from build123d import *

# Parameters (mm, degrees)
SKETCH1_W           = 300
SKETCH1_H           = 150
BOSS_EXTRUDE1_DEPTH = 5
SKETCH3_W           = 300
SKETCH3_H           = 150
SKETCH3_W_2         = 290
SKETCH3_H_2         = 140
BOSS_EXTRUDE2_DEPTH = 100
SKETCH4_W           = 290
SKETCH4_H           = 50
SKETCH4_H_2         = 60
BOSS_EXTRUDE3_DEPTH = 10
SKETCH7_R           = 12
CUT_EXTRUDE1_DEPTH  = 351
FILLET1_R           = 20
SKETCH10_W          = 180
SKETCH10_H          = 30
BOSS_EXTRUDE4_DEPTH = 15
SKETCH11_W          = 180
SKETCH11_H          = 30
BOSS_EXTRUDE5_DEPTH = 25
CHAMFER2_SIZE       = 15
CHAMFER3_SIZE       = 25
SKETCH12_W          = 133.404446906
SKETCH12_H          = 15
CUT_EXTRUDE2_DEPTH  = 50


with BuildPart() as part:
    # Sketch1 → Boss-Extrude1 (new body)
    with BuildSketch(Plane(origin=(0, 0, 0), x_dir=(1, 0, 0), z_dir=(0, 1, 0))):
        with Locations((150, 75)):
            Rectangle(SKETCH1_W, SKETCH1_H)
    extrude(amount=BOSS_EXTRUDE1_DEPTH)

    # Sketch3 → Boss-Extrude2 (add)
    with BuildSketch(Plane(origin=(0, 5, 0), x_dir=(1, 0, 0), z_dir=(0, 1, 0))):
        with Locations((150, 75)):
            Rectangle(SKETCH3_W, SKETCH3_H)
        with Locations((150, 75)):
            Rectangle(SKETCH3_W_2, SKETCH3_H_2, mode=Mode.SUBTRACT)
    extrude(amount=BOSS_EXTRUDE2_DEPTH)

    # Sketch4 → Boss-Extrude3 (add)
    with BuildSketch(Plane(origin=(0, 5, 0), x_dir=(1, 0, 0), z_dir=(0, 1, 0))):
        with Locations((150, 120)):
            Rectangle(SKETCH4_W, SKETCH4_H)
        with Locations((150, 35)):
            Rectangle(SKETCH4_W, SKETCH4_H_2)
    extrude(amount=BOSS_EXTRUDE3_DEPTH)

    # Sketch7 → Cut-Extrude1 (cut, through all)
    with BuildSketch(Plane(origin=(0, 5, 0), x_dir=(1, 0, 0), z_dir=(0, 1, 0))):
        with Locations(Location((150, 80, 0), (0, 0, 270))):
            Circle(SKETCH7_R)
    extrude(amount=-CUT_EXTRUDE1_DEPTH, mode=Mode.SUBTRACT)

    # Fillet1
    fillet1_edges = [part.edges().sort_by_distance(p)[0] for p in [
        (5, 60, -145),
        (5, 60, -5),
        (295, 60, -5),
        (295, 60, -145),
        (0, 52.5, -150),
        (300, 52.5, -150),
        (300, 52.5, 0),
        (0, 52.5, 0),
    ]]
    fillet(fillet1_edges, radius=FILLET1_R)

    # Sketch10 → Boss-Extrude4 (add)
    with BuildSketch(Plane.XY.offset(-145)):
        with Locations((150, 90)):
            Rectangle(SKETCH10_W, SKETCH10_H)
    extrude(amount=BOSS_EXTRUDE4_DEPTH)

    # Sketch11 → Boss-Extrude5 (add)
    with BuildSketch(Plane(origin=(0, 0, -5), x_dir=(-1, 0, 0), z_dir=(0, 0, -1))):
        with Locations((-150, 90)):
            Rectangle(SKETCH11_W, SKETCH11_H)
    extrude(amount=BOSS_EXTRUDE5_DEPTH)

    # Chamfer2
    chamfer2_edges = [part.edges().sort_by_distance(p)[0] for p in [
        (240, 90, -145),
        (150, 75, -145),
        (60, 90, -145),
    ]]
    chamfer(chamfer2_edges, length=CHAMFER2_SIZE - 0.0001)  # a hair under: the kernel refuses the full size

    # Chamfer3
    chamfer3_edges = [part.edges().sort_by_distance(p)[0] for p in [
        (60, 90, -5),
        (150, 75, -5),
        (240, 90, -5),
    ]]
    chamfer(chamfer3_edges, length=CHAMFER3_SIZE - 0.0001)  # a hair under: the kernel refuses the full size

    # Sketch12 → Cut-Extrude2 (cut)
    with BuildSketch(Plane(origin=(0, 105, 0), x_dir=(1, 0, 0), z_dir=(0, 1, 0))):
        with Locations((150, 7.5)):
            Rectangle(SKETCH12_W, SKETCH12_H)
    extrude(amount=-CUT_EXTRUDE2_DEPTH, mode=Mode.SUBTRACT)


solid = part.part
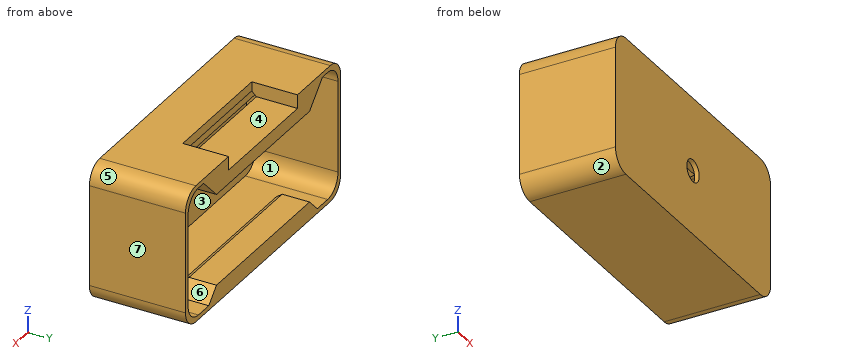
Source: CAD feature listing. Evaluate the final solid. Frame: model axes, mm. Face numbers are marked on the shaded views. A direction names the side the tool comes from. Round coordinates to 2 decimals unless told otherwise and drop trailing zeros. Write each loop counter-clockwise with the first axis right and the second up, starting at its lowest first coordinate (ties: lowest second). Pieces come first, ordered by that corner, then holes. Notation, with made-up numbers: (-20.75, 86.5) - (-2.75, 86.5) arc R7 cw to (-2.75, 98.5) - close; hole circle Ø3 at (-15.5, 40). An arc over 180 degrees is marked (long way). Use CSV: the item, a comma, the result in double quotes. Start each with the question number.
(1) Cut plane D-D, the plane y = 63.5. Return loops of the section in (x, z).
(2) Cut plane C-C, the plane z = -115. Return loops of the section in (x, y), and give its area (3 significant figures).
(3) First-contact query: pin 1 Ø22.5 at (x, y) = (131, 77.5) entering from +Z; pin 2 Ø25 at (x, z) = (102, -112.5) entering from +Y; pin 3 Ø4.5 at (y, z) = (86.5, -9) entering from +X. Flat tips, straight axial feed; report the tip coordinate or a pass-through.
(4) Mould query, pull axis Z, two halves, no side actions, for the marked faces 5, 6 and 7. Classes: pulls with the +Z half, pulls with the -Z half, needs draft (parallel to the pull), parting line crosses it, or undercut.
(5) Set-up query: the marked faces 1, 2, 3 and 4. Return all of +Z, -Z, +X, -X, +Y, -Y with unobstructed straight access to the full face (end or side cutting, diameter ignored); none if empty.
(6) Material intervals for probe 1 along Z at (x, y) = (92, 11.5); probe 2 along X at (y, z) = (98.5, -52); probe 3 along Z at (x, y) = (222, 88.5), sorted ascending. Write a range as [from, to].
(7) Cut plane A-A, the plane z = -80. Return loops of the section in (x, y), and give its area (3 significant figures).
(8) Cut plane B-B, the plane x = 150. Give the number of separate pieces and of enclosed holes in the cut face, and give its area (3 significant figures).
Geometry says:
1,outline,"(0, -130) arc R20 ccw to (20, -150) - (280, -150) arc R20 ccw to (300, -130) - (300, -20) arc R20 ccw to (280, 0) - (216.7, 0) - (216.7, -15) - (83.3, -15) - (83.3, 0) - (20, 0) arc R20 ccw to (0, -20) - close; hole (5, -125) arc R20 ccw to (25, -145) - (45, -145) - (48.5, -141.5) - (251.5, -141.5) - (255, -145) - (275, -145) arc R20 ccw to (295, -125) - (295, -25) arc R20 ccw to (275, -5) - (265, -5) - (251.5, -18.5) - (48.5, -18.5) - (35, -5) - (25, -5) arc R20 ccw to (5, -25) - close"
2,outline,"(0, 0) - (300, 0) - (300, 105) - (295, 105) - (295, 15) - (5, 15) - (5, 105) - (0, 105) - close"
2,area,"5,400 mm²"
3,pin 1,"z = -15"
3,pin 2,"y = 15"
3,pin 3,"x = 297.98"
4,face 5,"pulls with the +Z half"
4,face 6,"undercut"
4,face 7,"needs draft"
5,face 1,"+Y"
5,face 2,"-Z, -X, +Y, -Y"
5,face 3,"none"
5,face 4,"+Z, +Y"
6,probe 1,"[-150, -95], [-65, 0]"
6,probe 2,"[0, 5], [295, 300]"
6,probe 3,"[-150, -130], [-30, 0]"
7,outline,"(0, 0) - (138, 0) - (138, 5) - (5, 5) - (5, 105) - (0, 105) - close; (162, 0) - (300, 0) - (300, 105) - (295, 105) - (295, 5) - (162, 5) - close"
7,area,"2,380 mm²"
8,separate pieces,"3"
8,enclosed holes,"0"
8,area,"3,620 mm²"
